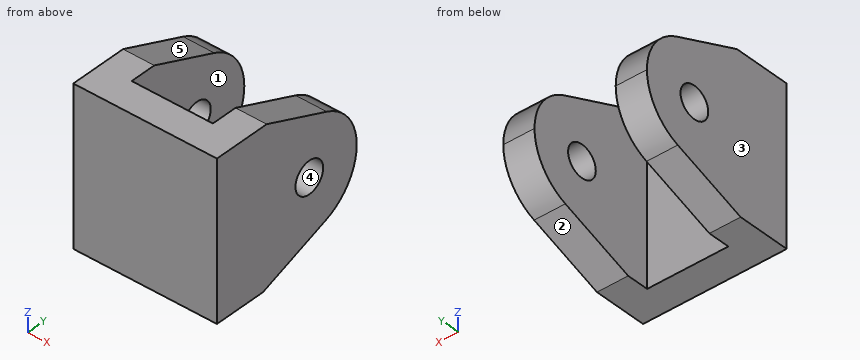
```python
from build123d import *

# Parameters (mm, degrees)
BOSS_EXTRUDE1_DEPTH    = 12.5
CUT_EXTRUDE1_START     = -11.5
CUT_EXTRUDE1_OUTLINE_R = 2.55
CUT_EXTRUDE1_DEPTH     = 23


# Read off the part's stored shape, not the designer's step: Cut-Extrude1
with BuildPart() as part:
    # Sketch1 → Boss-Extrude1 (new, symmetric)
    with BuildSketch(Plane.XY):
        Polygon((-6.5, 5), (6.5, 5), (6.5, 25.729927007), (11.5, 25.729927007), (11.5, 0), (-11.5, 0), (-11.5, 25.729927007), (-6.5, 25.729927007), align=None)
    extrude(amount=BOSS_EXTRUDE1_DEPTH, both=True)

    # Cut-Extrude1 outline → Cut-Extrude1 (cut)
    with BuildSketch(Plane(origin=(0, 0, 0), x_dir=(0, 0, -1), z_dir=(1, 0, 0)).offset(CUT_EXTRUDE1_START)):
        with BuildLine():
            Line((-12.5, 25.729927007), (-12.5, 9.159373111))
            Line((-12.5, 9.159373111), (-8.115271661, 20.217761866))
            ThreePointArc((-8.115271661, 20.217761866), (-4.905140127, 24.221580567), (0, 25.729927008))
            Line((0, 25.729927008), (-12.5, 25.729927007))
        make_face()
        with BuildLine():
            Line((12.5, 25.729927007), (0, 25.729927008))
            ThreePointArc((0, 25.729927008), (4.976994117, 24.172248959), (8.177901336, 20.055086791))
            Line((8.177901336, 20.055086791), (12.5, 8.485629403))
            Line((12.5, 8.485629403), (12.5, 25.729927007))
        make_face()
        with Locations((0, 17)):
            Circle(CUT_EXTRUDE1_OUTLINE_R)
    extrude(amount=CUT_EXTRUDE1_DEPTH, mode=Mode.SUBTRACT)


solid = part.part
```
The model under review builds one solid part; all positions refer to its coordinate system, in mm. Face numbers are marked on the shaded views. A direction names the side the tool comes from. Give positions to 0.01 mm unless a question says otherwise; leave off trailing zeros. Order: outer loops, then holes, each group sorted by start corner. A loop starts at its lowest first (then second) coordinate and runs counter-clockwise, first axis right, second up. Notation, with made-up numbers: (-5, 12) - (24, 12) arc R9 cw to (24, 25) - close; hole circle Ø9 at (28.25, 59). An arc over 180 degrees is marked (long way). Use CSV: the item, a comma, the result in double quotes. Start each with the question number.
Q1. To check wall thickness, follow line 1 along X through (y, z) = (11.75, -2.25); line 2 along Y through (x, z) = (-9.5, 0); line 3 along Y through (x, z) = (-0.75, -8.5). State the ranges of each line that lie inside material, in increasing order. Write a range as [from, to].
Q2. We need section A-A, the plane y = 17.75. Write out the cut boundary in (x, z), and give its area (3 significant figures).
Q3. We need section D-D, the plane y = 23. Write out the cut boundary in (x, z), and give its area (3 significant figures).
Q4. Clearance check with flat-ended pins moving along their axes: pin 1 Ø5 at (x, z) = (6.5, -7.5) entering from +Y; pin 2 Ø1.5 at (x, y) = (-5.5, 22) entering from -Z; pin 3 Ø10.5 at (x, z) = (2, -3) entering from +Y. State where each tip first meets the part, or that it passes through.
Q5. We need section B-B, the plane x = 9. Write out the cut boundary in (y, z), and give its area (3 significant figures).
Q6. The part is to be moulded in two halves that separate along Z. For the marked faces 3, 4 and 5, say which applies: +Z half, -Z half, draft (parallel to the pull), parting line (faces both ways), or undercut.
Q7. We need section C-C, the plane z = 1.5. Write out the cut boundary in (x, y).
Q8. Tool access review of the marked faces 1 and 2: name each direction out of +Z, -Z, +X, -X, +Y, -Y from which nothing blocks a thin tool from reaching the whole face with its end or side.
Outcome:
1,line 1,"x = [-11.5, -6.5], [6.5, 11.5]"
1,line 2,"y = [0, 14.45], [19.55, 25.73]"
1,line 3,"y = [0, 5]"
2,outline,"(-11.5, -9.04) - (-6.5, -9.04) - (-6.5, -2.44) - (-11.5, -2.44) - close; (-11.5, 2.44) - (-6.5, 2.44) - (-6.5, 9.09) - (-11.5, 9.09) - close; (6.5, -9.04) - (11.5, -9.04) - (11.5, -2.44) - (6.5, -2.44) - close; (6.5, 2.44) - (11.5, 2.44) - (11.5, 9.09) - (6.5, 9.09) - close"
2,area,"133 mm^2"
3,outline,"(-11.5, -6.34) - (-6.5, -6.34) - (-6.5, 6.34) - (-11.5, 6.34) - close; (6.5, -6.34) - (11.5, -6.34) - (11.5, 6.34) - (6.5, 6.34) - close"
3,area,"127 mm^2"
4,pin 1,"stops at y = 24.16"
4,pin 2,"passes through"
4,pin 3,"stops at y = 25.72"
5,outline,"(0, -12.5) - (8.49, -12.5) - (20.06, -8.18) arc R8.73 ccw to (20.22, 8.12) - (9.16, 12.5) - (0, 12.5) - close; hole circle Ø5.1 at (17, 0)"
5,area,"500 mm^2"
6,face 3,"draft"
6,face 4,"undercut"
6,face 5,"+Z half"
7,outline,"(-11.5, 0) - (11.5, 0) - (11.5, 14.94) - (6.5, 14.94) - (6.5, 5) - (-6.5, 5) - (-6.5, 14.94) - (-11.5, 14.94) - close; (-11.5, 19.06) - (-6.5, 19.06) - (-6.5, 25.6) - (-11.5, 25.6) - close; (6.5, 19.06) - (11.5, 19.06) - (11.5, 25.6) - (6.5, 25.6) - close"
8,face 1,"+Z, -Z, +Y"
8,face 2,"-Z, +X, -X, +Y"
